from build123d import *

# Parameters (mm, degrees)
BOSS_EXTRU_1_DEPTH      = 0.5
ESQUISSE2_R             = 7.25
ESQUISSE2_R_2           = 7
BOSS_EXTRU_2_DEPTH      = 8
D_GAGEMENT_M21_D        = 2.4
D_GAGEMENT_M21_DEPTH    = 10
D_GAGEMENT_M21_TIP      = 0.721032743
ESQUISSE16_R            = 7.25
BOSS_EXTRU_4_DEPTH      = 0.75
ESQUISSE7_R             = 0.75
ENL_V_MAT_EXTRU_1_DEPTH = 18.396120257


with BuildPart() as part:
    # Esquisse1 → Boss.-Extru.1 (new body)
    with BuildSketch(Plane.XY):
        with BuildLine():
            Line((-11.125, 1.948557159), (-3.625, 6.278684177))
            ThreePointArc((-3.625, 6.278684177), (0, 7.25), (3.625, 6.278684177))
            Line((3.625, 6.278684177), (11.125, 1.948557159))
            ThreePointArc((11.125, 1.948557159), (12.25, 0), (11.125, -1.948557159))
            Line((11.125, -1.948557159), (3.625, -6.278684177))
            ThreePointArc((3.625, -6.278684177), (0, -7.25), (-3.625, -6.278684177))
            Line((-3.625, -6.278684177), (-11.125, -1.948557159))
            ThreePointArc((-11.125, -1.948557159), (-12.25, 0), (-11.125, 1.948557159))
        make_face()
    extrude(amount=BOSS_EXTRU_1_DEPTH)

    # Esquisse2 → Boss.-Extru.2 (add)
    with BuildSketch(Plane.XY.offset(0.5)):
        with Locations(Location((0, 0, 0), (0, 0, 120))):
            Circle(ESQUISSE2_R)
        Circle(ESQUISSE2_R_2, mode=Mode.SUBTRACT)
    extrude(amount=BOSS_EXTRU_2_DEPTH)

    # Dégagement M21
    with Locations(Plane(origin=(-10, 0, 0.5), x_dir=(1, 0, 0), z_dir=(0, 0, 1))):
        with Locations((0, 0), (20, 0)):
            Hole(D_GAGEMENT_M21_D / 2, depth=D_GAGEMENT_M21_DEPTH)
            with Locations((0, 0, -(D_GAGEMENT_M21_DEPTH + D_GAGEMENT_M21_TIP / 2))):  # 118° drill point
                Cone(0, D_GAGEMENT_M21_D / 2, D_GAGEMENT_M21_TIP, mode=Mode.SUBTRACT)



with BuildPart() as body_2:
    # Esquisse5 → Révolution1 (revolve)
    with BuildSketch(Plane(origin=(0, 0, 0), x_dir=(1, 0, 0), z_dir=(0, 1, 0))):
        Polygon((-6, -9.25), (-6, -9.5), (-3, -9.5), (-3, -10), (-0.75, -10), (-0.75, -9.25), align=None)
    revolve(axis=Axis((0, 0, 0), (0, 0, 1)))


with BuildPart() as part_1:
    add(part.part)

    add(body_2.part)  # Boss.-Extru.4 merges body 2
    # Esquisse16 → Boss.-Extru.4 (add)
    with BuildSketch(Plane.XY.offset(8.5)):
        with Locations(Location((0, 0, 0), (0, 0, 180))):
            Circle(ESQUISSE16_R)
    extrude(amount=BOSS_EXTRU_4_DEPTH)

    # Esquisse7 → Enlèv. mat.-Extru.1 (cut, through all)
    with BuildSketch(Plane(origin=(0, 0, 0), x_dir=(-1, 0, 0), z_dir=(0, 0, -1))):
        Circle(ESQUISSE7_R)
    extrude(amount=-ENL_V_MAT_EXTRU_1_DEPTH, mode=Mode.SUBTRACT)


solid = part_1.part
Could you check a few things on this model? Use its own coordinates, in mm. A direction names the side the tool comes from. Give positions to 0.01 mm unless a question says otherwise; leave off trailing zeros. Write each loop counter-clockwise with the first axis right and the second up, starting at its lowest first coordinate (ties: lowest second). Pieces come first, ordered by that corner, then holes. Notation, with made-up numbers: (51, -21.5) -> (57, -21.5) arc R19 ccw to (57, 9.5) -> close; hole circle Ø7 at (70.25, -16). An arc over 180 degrees is marked (long way). Write each question's results on one line, items separated by ' | '. Start each with the question number.
Q1. Suppose I cut it at D-D, the plane y = 0. State how many separate pieces and enclosed holes the cut face has, and give its area (3 significant figures).
Q2. Suppose I cut it at A-A, the plane x = 0. List the corners of the cut face in (y, z) for me, and give its area (3 significant figures).
Q3. Which directions (+Z, -Z, +X, -X, +Y, -Y) give clear straight access to the entire face, cutting with the end or side of a thin tool? Please do faces 1 (the face through (3, -0.1, 9.8)), 2 (the face through (-1, 0, 8.5)), 3 (the face through (12.25, 0.03, 0.25)).
Q4. I need wall thicknesses on probe 1 along Z at (x, y) = (1.75, 6.5); probe 2 along X at (y, z) = (0, 9.75); probe 3 along Z at (x, y) = (-3, 1.5). Which ranges of each line are inside material? Lowest first, please.
Q5. Suppose I cut it at C-C, the plane x = 4.25. List the corners of the cut face in (y, z) for me.
Q6. I'm going to push flat-ended pins straight in: pin 1 Ø6 at (x, z) = (8.5, 4.5) entering from -Y; pin 2 Ø3 at (x, y) = (-10, 0) entering from +Z; pin 3 Ø5 at (x, z) = (-6, 4.5) entering from +Y; pin 4 Ø1.2 at (x, y) = (0, 0) entering from +Z. Where does each tip first touch, or does it pass through?
Q7. We'd pull the mould along Z, two halves only. Please class faces 4 (the face through (-12.25, -0.03, 0.25)), 5 (the face through (0, 2, 0)), 6 (the face through (6.466, -2.681, 4.444)): +Z half, -Z half, draft (parallel to the pull), parting line (faces both ways), or undercut.
Q8. Suppose I cut it at B-B, the plane y = 3.75. List the corners of the cut face in (x, z) for me.
Outcome:
1) separate pieces: 4 | enclosed holes: 0 | area: 27.7 mm2
2) outline: (-7.25, 0) -> (-0.75, 0) -> (-0.75, 0.5) -> (-7, 0.5) -> (-7, 8.5) -> (-0.75, 8.5) -> (-0.75, 10) -> (-3, 10) -> (-3, 9.5) -> (-6, 9.5) -> (-6, 9.25) -> (-7.25, 9.25) -> close; (0.75, 0) -> (7.25, 0) -> (7.25, 9.25) -> (6, 9.25) -> (6, 9.5) -> (3, 9.5) -> (3, 10) -> (0.75, 10) -> (0.75, 8.5) -> (7, 8.5) -> (7, 0.5) -> (0.75, 0.5) -> close | area: 25.1 mm2
3) face 1: +Z | face 2: none | face 3: +Z, -Z, +X
4) probe 1: 0 to 0.5, 8.5 to 9.25 | probe 2: -3 to -0.75, 0.75 to 3 | probe 3: 0 to 0.5, 8.5 to 9.5
5) outline: (-5.92, 0) -> (5.92, 0) -> (5.92, 0.5) -> (5.87, 0.5) -> (5.87, 9.25) -> (4.24, 9.25) -> (4.24, 9.5) -> (-4.24, 9.5) -> (-4.24, 9.25) -> (-5.87, 9.25) -> (-5.87, 0.5) -> (-5.92, 0.5) -> close; hole (-5.56, 0.5) -> (5.56, 0.5) -> (5.56, 8.5) -> (-5.56, 8.5) -> close
6) pin 1: y = -4.72 | pin 2: z = 0.5 | pin 3: y = 6.35 | pin 4: through
7) face 4: draft | face 5: -Z half | face 6: undercut
8) outline: (-8, 0) -> (8, 0) -> (8, 0.5) -> (6.2, 0.5) -> (6.2, 9.25) -> (4.68, 9.25) -> (4.68, 9.5) -> (-4.68, 9.5) -> (-4.68, 9.25) -> (-6.2, 9.25) -> (-6.2, 0.5) -> (-8, 0.5) -> close; hole (-5.91, 0.5) -> (5.91, 0.5) -> (5.91, 8.5) -> (-5.91, 8.5) -> close
